from build123d import *

# Parameters (mm, degrees)
BOSS_EXTRUDE1_DEPTH       = 3.175
F_8_CLEARANCE_HOLE1_D     = 4.9149
F_8_CLEARANCE_HOLE1_DEPTH = 3.175


with BuildPart() as part:
    # Sketch1 → Boss-Extrude1 (new body)
    with BuildSketch(Plane.XY):
        Polygon((-829.363556946, 6406.612895041), (-975.413556946, 6406.612895041), (-975.413556946, 6641.646276193), (-829.363556946, 6632.389598842), align=None)
    extrude(amount=BOSS_EXTRUDE1_DEPTH)

    # #8 Clearance Hole1
    with Locations(Plane.XY.offset(3.175)):
        with Locations((-970.524056946, 6609.812895041), (-970.524056946, 6562.187895041), (-970.524056946, 6514.562895041), (-970.524056946, 6466.937895041), (-970.524056946, 6419.312895041), (-834.126056946, 6419.312895041), (-834.126056946, 6466.937895041), (-834.126056946, 6514.562895041), (-834.126056946, 6562.187895041), (-834.126056946, 6609.812895041)):
            Hole(F_8_CLEARANCE_HOLE1_D / 2, depth=F_8_CLEARANCE_HOLE1_DEPTH)


solid = part.part
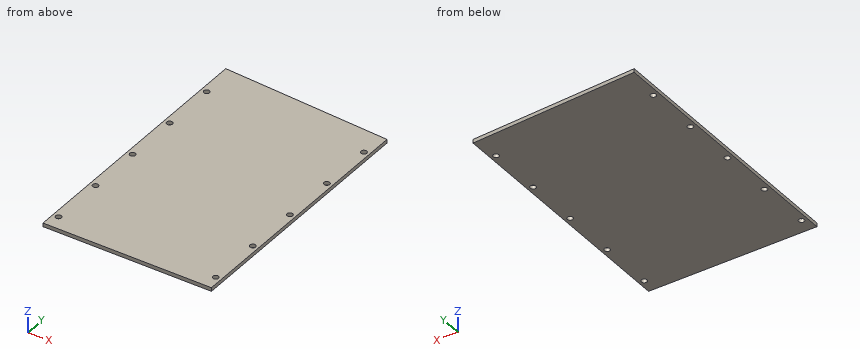
Source: CAD feature listing. Evaluate the final solid. Frame: model axes, mm. Coordinates: 2 decimals unless noted, no trailing zeros. Loops run counter-clockwise (first coordinate to the right, second up) from the corner with the lowest first, then second, coordinate; pieces in that order, holes last. Notation, with made-up numbers: (19, 25) - (77, 25) arc R24 ccw to (77, 44) - close; hole circle Ø11 at (43, 43). An arc over 180 degrees is marked (long way). One line per question, with ' | ' between items.
1) Section B-B, the plane x = -914.5. Return loops of the section in (y, z) (3 decimals).
Report:
outline: (6406.613, 0) - (6637.786, 0) - (6637.786, 3.175) - (6406.613, 3.175) - close
2) First-contact query: P1, Ø4.5, axis at x = -970.52, y = 6514.56, coming from the +Z side; P2, Ø8, axis at x = -834.13, y = 6514.56, coming from the -Z side. Flat tips, straight axial feed; report the tip coordinate or a pass-through.
Report:
P1: passes through | P2: stops at z = 0
3) Section C-C, the plane x = -878. Return loops of the section in (y, z) (3 decimals), then the cut area to 3 significant figures.
Report:
outline: (6406.613, 0) - (6635.472, 0) - (6635.472, 3.175) - (6406.613, 3.175) - close | area: 727 mm²
4) Section A-A, the plane z = 0.55. Give the number of separate pieces and of enclosed holes in the cut face, then the cut area to 3 significant figures.
Report:
separate pieces: 1 | enclosed holes: 10 | area: 33,500 mm²
5) Line query: line 1 along Y through (x, z) = (-902, 1.25); line 2 along Y through (x, z) = (-936.5, 0.9). Output: solid intervals per line, ascending.
Report:
line 1: y = 6406.61 to 6636.99 | line 2: y = 6406.61 to 6639.18
